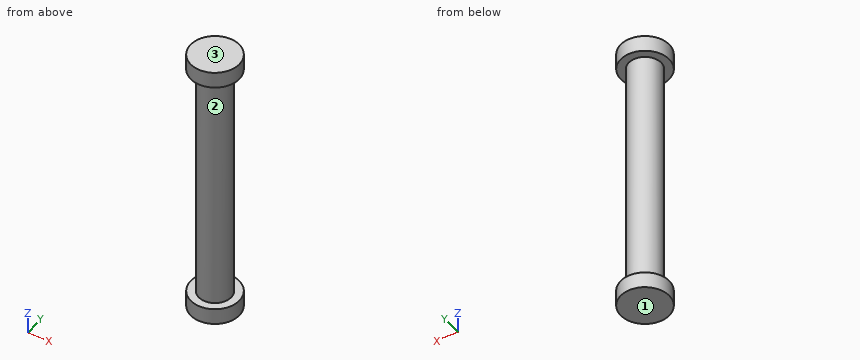
```python
from build123d import *

# Parameters (mm, degrees)
SKETCH1_R           = 6.35
BOSS_EXTRUDE1_DEPTH = 95.25
SKETCH2_R           = 9.525
BOSS_EXTRUDE2_DEPTH = 6.35
SKETCH3_R           = 9.525
BOSS_EXTRUDE3_DEPTH = 6.35


with BuildPart() as part:
    # Sketch1 → Boss-Extrude1 (new body)
    with BuildSketch(Plane.XY):
        Circle(SKETCH1_R)
    extrude(amount=-BOSS_EXTRUDE1_DEPTH)

    # Sketch2 → Boss-Extrude2 (add)
    with BuildSketch(Plane.XY):
        Circle(SKETCH2_R)
    extrude(amount=BOSS_EXTRUDE2_DEPTH)

    # Sketch3 → Boss-Extrude3 (add)
    with BuildSketch(Plane(origin=(0, 0, -95.25), x_dir=(-1, 0, 0), z_dir=(0, 0, -1))):
        Circle(SKETCH3_R)
    extrude(amount=BOSS_EXTRUDE3_DEPTH)


solid = part.part
```
CAD build for the part. Positions are in the model's coordinates, mm. Face numbers are marked on the shaded views. Round coordinates to 2 decimals unless told otherwise and drop trailing zeros. Loops run counter-clockwise (first coordinate to the right, second up) from the corner with the lowest first, then second, coordinate; pieces in that order, holes last. Notation, with made-up numbers: (-21.75, -3.5) - (15.25, -3.5) arc R26 ccw to (15.25, 26.5) - close; hole circle Ø4 at (-32.75, 82.5). An arc over 180 degrees is marked (long way). Return JSON: item names as keys, results as strings. Group by question number.
Q1. Flat gauge pins, fed straight in: pin 1 Ø10 at (x, z) = (6.5, -53) entering from +Y; pin 2 Ø1 at (y, z) = (-2.5, -16) entering from +X; pin 3 Ø3 at (y, z) = (4, -34) entering from -X. Where does each tip first touch, or does it go through?
Q2. Band-saw the part on A-A on x = 0. Give the cut face in (y, z) (3 decimals).
Q3. Band-saw the part on D-D on z = -68. Give the cut face in (x, y), plus the area to 3 significant figures.
Q4. Two-plate mould, pull along Z, no slides. Class the marked faces 1, 2 and 3: +Z half, -Z half, draft (parallel to the pull), parting line (faces both ways), or undercut.
Q5. Band-saw the part on B-B on y = 7.75. Give the cut face in (x, z).
Q6. Drill centre lines: line 1 along Z through (x, y) = (2.25, -6.5); line 2 along X through (y, z) = (0.5, -62.5). Where is each one in solid material? Low to high. Write a range as [from, to].
Solutions:
{
 "1": {"pin 1": "stops at y = 6.17", "pin 2": "stops at x = 6.03", "pin 3": "stops at x = -5.84"},
 "2": {"outline": "(-9.525, -101.6) - (9.525, -101.6) - (9.525, -95.25) - (6.35, -95.25) - (6.35, 0) - (9.525, 0) - (9.525, 6.35) - (-9.525, 6.35) - (-9.525, 0) - (-6.35, 0) - (-6.35, -95.25) - (-9.525, -95.25) - close"},
 "3": {"outline": "circle Ø12.7 at (0, 0)", "area": "127 mm^2"},
 "4": {"face 1": "-Z half", "face 2": "undercut", "face 3": "+Z half"},
 "5": {"outline": "(-5.54, -101.6) - (5.54, -101.6) - (5.54, -95.25) - (-5.54, -95.25) - close; (-5.54, 0) - (5.54, 0) - (5.54, 6.35) - (-5.54, 6.35) - close"},
 "6": {"line 1": "z = [-101.6, -95.25], [0, 6.35]", "line 2": "x = [-6.33, 6.33]"}
}
